Design review of the part shown in the three views and the two pictorial views. Dimensions are in mm from the part's minimum x, y and z. A direction names the side the tool comes from. Round coordinates to 2 decimals unless told otherwise and drop trailing zeros. Write each loop counter-clockwise with the first axis right and the second up, starting at its lowest first coordinate (ties: lowest second). Pieces come first, ordered by that corner, then holes. Notation, with made-up numbers: (-2, 47.25) -> (48, 47.25) arc R17 cw to (48, 75.25) -> close; hole circle Ø1 at (-15, -15). An arc over 180 degrees is marked (long way). One line per question, with ' | ' between items. Start each with the question number.
1) For probe 1 along Z at (x, y) = (253, 118.5); probe 2 along X at (y, z) = (131.5, 119.5); probe 3 along X at (y, z) = (187.5, 84.5), list the stretches that pass through material, from the lowest coordinate up.
2) Consider section C-C (x = 61). Give the boundary of the cut face in (y, z).
3) For the marked faces 1, 2, 3, 4 and 5, list the 3-axis set-ups (+Z, -Z, +X, -X, +Y, -Y) from which the entire face can be reached by the end or side of a thin tool; tool diameter is ignored.
4) Insertion check: pin 1 Ø6 at (y, z) = (47, 91) entering from -X; pin 2 Ø8 at (y, z) = (25, 65.5) entering from +X. Each pin has a flat end and moves straight along its axis. Give the tip position at first contact, or say it passes through.
5) Consider section B-B (y = 161.5). Give the boundary of the cut face in (x, z).
6) Consider section D-D (x = 256.5). Give the boundary of the cut face in (y, z).
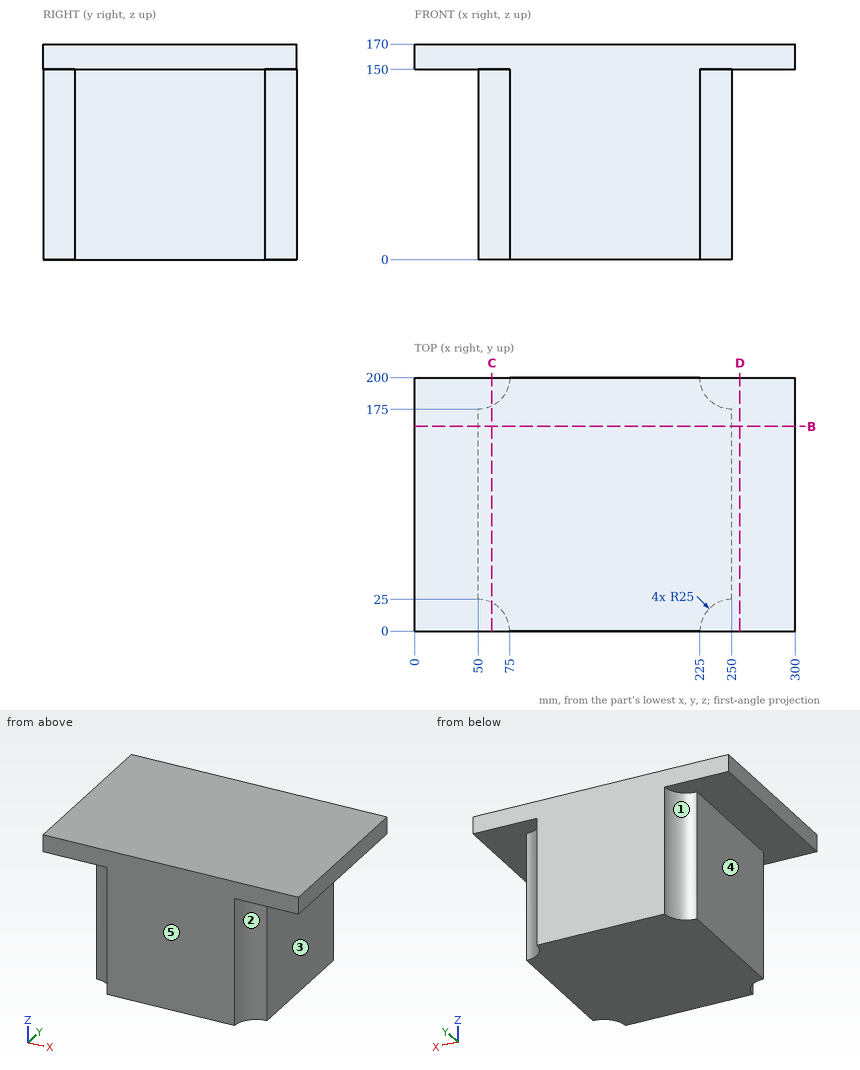
From the geometry:
1) probe 1: z = 150 to 170 | probe 2: x = 50 to 250 | probe 3: x = 71.65 to 228.35
2) outline: (0, 150) -> (22.45, 150) -> (22.45, 0) -> (177.55, 0) -> (177.55, 150) -> (200, 150) -> (200, 170) -> (0, 170) -> close
3) face 1: -Z, -X, +Y | face 2: -Z, +X, -Y | face 3: -Z, +X, +Y, -Y | face 4: -Z, -X, +Y, -Y | face 5: +Z, -Z, +X, -X, -Y
4) pin 1: stops at x = 50 | pin 2: stops at x = 250
5) outline: (0, 150) -> (50, 150) -> (50, 0) -> (250, 0) -> (250, 150) -> (300, 150) -> (300, 170) -> (0, 170) -> close
6) outline: (0, 150) -> (200, 150) -> (200, 170) -> (0, 170) -> close
